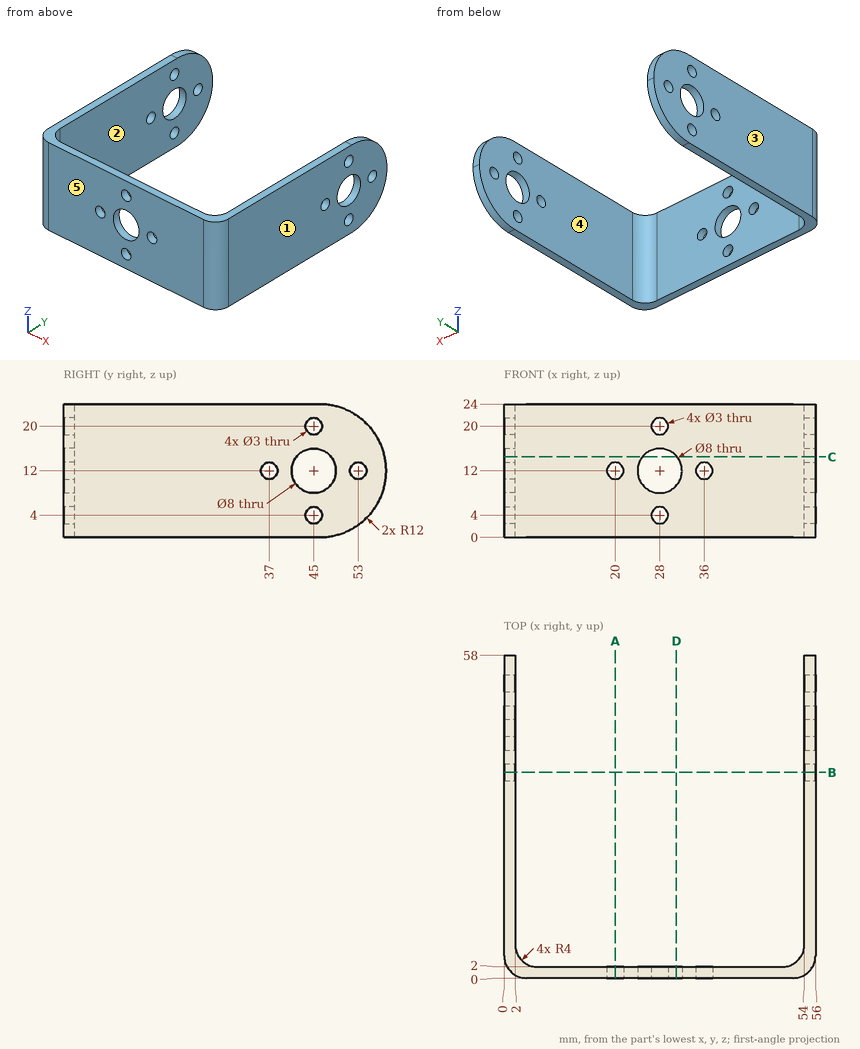
Source: three-view drawing plus pictorial views. Frame: mm from the lowest corner of the part. A direction names the side the tool comes from. Round coordinates to 2 decimals unless told otherwise and drop trailing zeros. Loops run counter-clockwise (first coordinate to the right, second up) from the corner with the lowest first, then second, coordinate; pieces in that order, holes last. Notation, with made-up numbers: (79.5, 77.5) - (103.5, 77.5) arc R22 ccw to (103.5, 92.5) - close; hole circle Ø3 at (-29, 87.5). An arc over 180 degrees is marked (long way). Write each question's results on one line, items separated by ' | '. Start each with the question number.
1) First-contact query: P1, Ø4, axis at x = 42.5, z = 10, coming from the +Y side. Flat tip, straight axial feed; report the tip coordinate or a pass-through.
2) Cut plane A-A on x = 20. Return loops of the section in (y, z), then the cut area to 3 significant figures.
3) Access query for the marked faces 4 and 5. Directions: +Z, -Z, +X, -X, +Y, -Y. A direction counts if a zero-diameter tool reaches every point of the face in a straight line with its end or side. Return the directions, or none.
4) Cut plane C-C on z = 14.5. Return loops of the section in (x, y).
5) Cut plane B-B on y = 37. Return loops of the section in (x, z).
6) Line query: probe 1 along Z at (x, y) = (0.5, 45); probe 2 along X at (y, z) = (13, 1); probe 3 along Z at (x, y) = (36, 0.7). Output: solid intervals per line, ascending. Write a range as [from, to].
7) Cut plane D-D on x = 31. Return loops of the section in (y, z), then the cut area to 3 significant figures.
8) Mould query, pull axis X, two halves, no side actions, for the marked faces 1, 2 and 3. Classes: released by +X, released by -X, zero draft, split by the parting line, or undercut.
Verdict:
1) P1: stops at y = 2
2) outline: (0, 0) - (2, 0) - (2, 10.5) - (0, 10.5) - close; (0, 13.5) - (2, 13.5) - (2, 24) - (0, 24) - close | area: 42.0 mm2
3) face 4: +Z, -Z, +Y | face 5: +Z, -Z, +X, -X, -Y
4) outline: (0, 4) arc R4 ccw to (4, 0) - (24.88, 0) - (24.88, 2) - (6, 2) arc R4 cw to (2, 6) - (2, 41.88) - (0, 41.88) - close; (0, 48.12) - (2, 48.12) - (2, 57.74) - (0, 57.74) - close; (31.12, 0) - (52, 0) arc R4 ccw to (56, 4) - (56, 41.88) - (54, 41.88) - (54, 6) arc R4 cw to (50, 2) - (31.12, 2) - close; (54, 48.12) - (56, 48.12) - (56, 57.74) - (54, 57.74) - close
5) outline: (0, 0) - (2, 0) - (2, 10.5) - (0, 10.5) - close; (0, 13.5) - (2, 13.5) - (2, 24) - (0, 24) - close; (54, 0) - (56, 0) - (56, 10.5) - (54, 10.5) - close; (54, 13.5) - (56, 13.5) - (56, 24) - (54, 24) - close
6) probe 1: z = [0, 2.5], [5.5, 8], [16, 18.5], [21.5, 24] | probe 2: x = [0, 2], [54, 56] | probe 3: z = [0, 10.5], [13.5, 24]
7) outline: (0, 0) - (2, 0) - (2, 9.35) - (0, 9.35) - close; (0, 14.65) - (2, 14.65) - (2, 24) - (0, 24) - close | area: 37.4 mm2
8) face 1: released by +X | face 2: undercut | face 3: released by -X
